Source: three-view drawing plus pictorial views. Frame: mm from the lowest corner of the part. Round coordinates to 2 decimals unless told otherwise and drop trailing zeros. Loops run counter-clockwise (first coordinate to the right, second up) from the corner with the lowest first, then second, coordinate; pieces in that order, holes last. Notation, with made-up numbers: (17.5, 43) -> (21.5, 43) arc R20 cw to (21.5, 64) -> close; hole circle Ø4 at (-8.5, 23.25). An arc over 180 degrees is marked (long way). Answer in a Markdown table with one row per item.
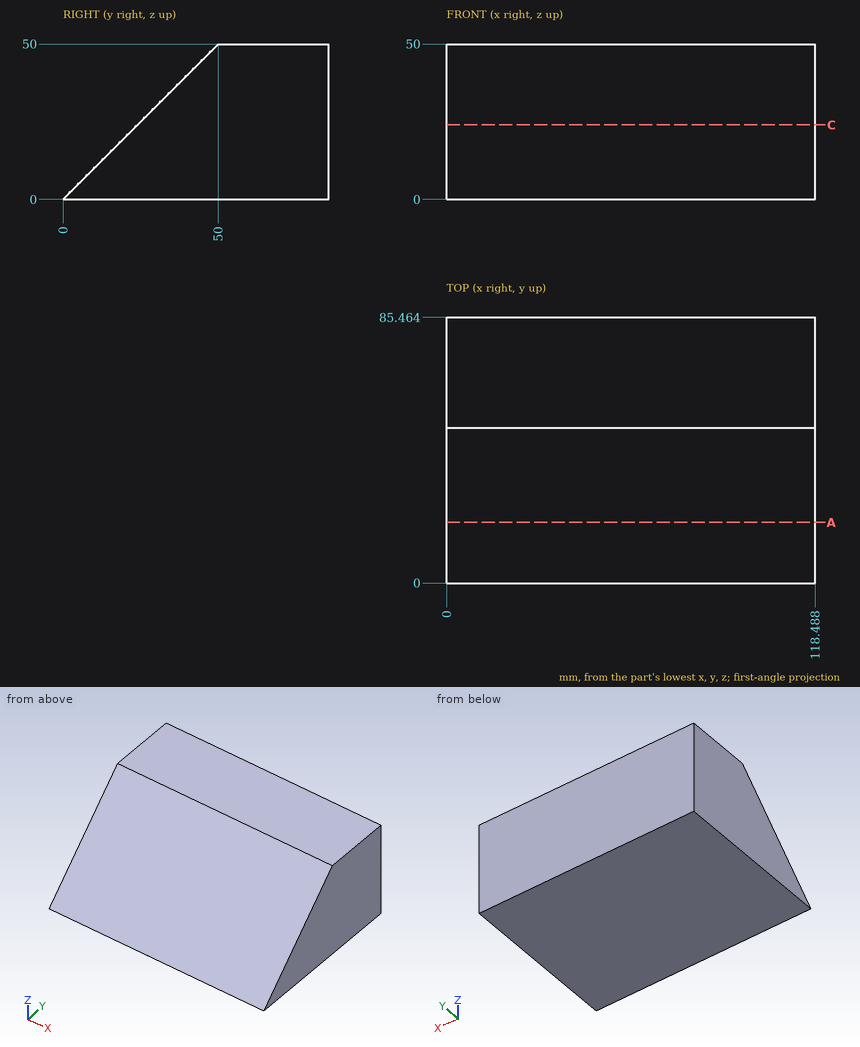
Item 1: Pin query (flat end, axial travel): pin 1 Ø1.5 at (x, z) = (34.5, 23.5) entering from -Y; pin 2 Ø12 at (x, y) = (18, 26) entering from +Z; pin 3 Ø1 at (x, z) = (102.5, 39.5) entering from -Y. Return the tip coordinate at first contact, or that it passes through.
Answer:
| item | result |
|---|---|
| pin 1 | stops at y = 22.75 |
| pin 2 | stops at z = 32 |
| pin 3 | stops at y = 39 |
Item 2: Cut plane A-A (y = 19.5). Output: boundary loops of the cut face in (x, z), then the cut area to 3 significant figures.
Answer:
| item | result |
|---|---|
| outline | (0, 0) -> (118.49, 0) -> (118.49, 19.5) -> (0, 19.5) -> close |
| area | 2,310 mm² |
Item 3: Cut plane C-C (z = 24). Output: boundary loops of the cut face in (x, y), then the cut area to 3 significant figures.
Answer:
| item | result |
|---|---|
| outline | (0, 24) -> (118.49, 24) -> (118.49, 85.46) -> (0, 85.46) -> close |
| area | 7,280 mm² |
Item 4: Line query: probe 1 along Z at (x, y) = (106.5, 14.5); probe 2 along Y at (x, z) = (46.5, 5) (1 decimal); probe 3 along Y at (x, z) = (71.5, 10) (1 decimal). Output: solid intervals per line, ascending. Write a range as [from, to].
Answer:
| item | result |
|---|---|
| probe 1 | z = [0, 14.5] |
| probe 2 | y = [5, 85.5] |
| probe 3 | y = [10, 85.5] |
